Read the model definition and answer for the solid it produces. Units are mm, in the model's axes. Face numbers are marked on the shaded views. A direction names the side the tool comes from. Round coordinates to 2 decimals unless told otherwise and drop trailing zeros. Order: outer loops, then holes, each group sorted by start corner. A loop starts at its lowest first (then second) coordinate and runs counter-clockwise, first axis right, second up. Notation, with made-up numbers: (22.25, 2.25) -> (54.25, 2.25) arc R21 ccw to (54.25, 23.25) -> close; hole circle Ø9 at (16.5, -2). An arc over 180 degrees is marked (long way). Answer as a JSON object with one key per item and string values. Group by question number.
Item 1: Section C-C, the plane y = 215.5 is taken. Write down the section's boundary in (x, z).
Item 2: The mould has two halves that part along Y. Classify the marked faces 1, 2 and 3: pulls with the +Y half, pulls with the -Y half, needs draft (parallel to the pull), parting line crosses it, or undercut.
Item 3: Consider probe 1 along Y at (x, z) = (-66, 7); probe 2 along Z at (x, y) = (-131, 194); probe 3 along Y at (x, z) = (-16, 16.5). Determine where each line is inside the solid, lowest interval first. Write a range as from..to.
Item 4: Given P1, Ø3, axis at x = 66.5, y = 186, coming from the +Z side; P2, Ø8, axis at x = -114, z = 26, coming from the +Y side; P3, Ø10, axis at x = -110.5, z = 7.5, coming from the -Y side, each flat-ended and moving along its own axis, determine where each tip first touches the part or whether it passes through.
Item 5: Section A-A, the plane z = 15 is taken. Count the separate pieces of the cut face and the enclosed holes in it, plus the area to 3 significant figures.
Item 6: For the marked faces 4, 5, 6 and 7, determine the directions among +Z, -Z, +X, -X, +Y, -Y from which every point of the face is accessible in a straight line to the end or side of a thin tool.
Item 7: Section B-B, the plane x = -80.5 is taken. Write down the section's boundary in (y, z), plus the area to 3 significant figures.
Item 8: Section D-D, the plane x = 43.5 is taken. Write down the section's boundary in (y, z).
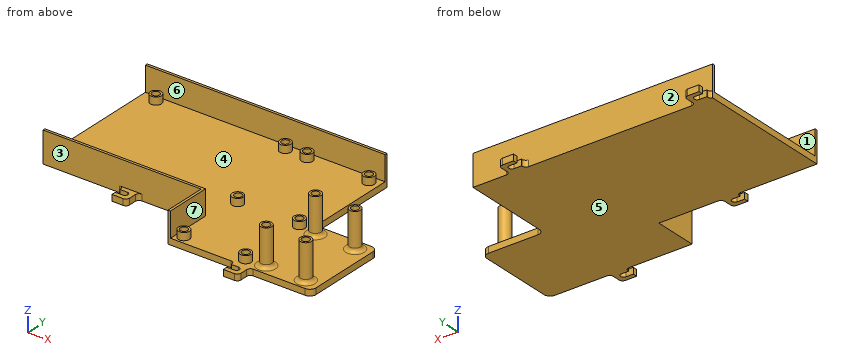
from build123d import *

# Parameters (mm, degrees)
SKETCH1_W            = 128
SKETCH1_H            = 110
SKETCH1_W_2          = 50
SKETCH1_H_2          = 70
BOSS_EXTRUDE1_DEPTH  = 5
SKETCH3_W            = 128
SKETCH3_H            = 2
SKETCH3_W_2          = 194
BOSS_EXTRUDE3_DEPTH  = 20
SKETCH6_W            = 12
SKETCH6_H            = 12
BOSS_EXTRUDE5_DEPTH  = 5
M4_CLEARANCE_HOLE1_D = 4.8
CUT_EXTRUDE1_DEPTH   = 329.83563266
FILLET2_R            = 3
FILLET3_R            = 5
SKETCH15_R           = 4.5
SKETCH15_R_2         = 3.025
BOSS_EXTRUDE6_DEPTH  = 6
SKETCH16_R           = 4.5
SKETCH16_R_2         = 3.025
BOSS_EXTRUDE7_DEPTH  = 30
FILLET4_R            = 3


with BuildPart() as part:
    # Sketch1 → Boss-Extrude1 (new body)
    with BuildSketch(Plane.XY):
        with Locations((-103.32475602, 215.37439567)):
            Rectangle(SKETCH1_W, SKETCH1_H)
        Polygon((26.67524398, 270.37439567), (-39.32475602, 270.37439567), (-39.32475602, 160.37439567), (-39.32475602, 125.37439567), (26.67524398, 125.37439567), (26.67524398, 195.37439567), align=None)
        with Locations((51.67524398, 160.37439567)):
            Rectangle(SKETCH1_W_2, SKETCH1_H_2)
    extrude(amount=BOSS_EXTRUDE1_DEPTH)

    # Sketch3 → Boss-Extrude3 (add)
    with BuildSketch(Plane.XY.offset(5)):
        Polygon((-37.32475602, 162.37439567), (-39.32475602, 162.37439567), (-39.32475602, 160.37439567), (-39.32475602, 125.37439567), (-37.32475602, 125.37439567), align=None)
        with Locations((-103.32475602, 161.37439567)):
            Rectangle(SKETCH3_W, SKETCH3_H)
        with Locations((-70.32475602, 269.37439567)):
            Rectangle(SKETCH3_W_2, SKETCH3_H)
    extrude(amount=BOSS_EXTRUDE3_DEPTH)

    # Sketch6 → Boss-Extrude5 (add)
    with BuildSketch(Plane(origin=(0, 0, 0), x_dir=(-1, 0, 0), z_dir=(0, 0, -1))):
        with Locations((96.32475602, 154.37439567)):
            Rectangle(SKETCH6_W, SKETCH6_H)
        with Locations((159.32475602, 276.37439567)):
            Rectangle(SKETCH6_W, SKETCH6_H)
        with Locations((-20.67524398, 119.37439567)):
            Rectangle(SKETCH6_W, SKETCH6_H)
        with Locations((9.32475602, 276.37439567)):
            Rectangle(SKETCH6_W, SKETCH6_H)
    extrude(amount=-BOSS_EXTRUDE5_DEPTH)

    # M4 Clearance Hole1 (through all)
    with Locations(Plane.XY.offset(5)):
        with Locations((-96.32475602, 154.37439567), (-159.32475602, 276.37439567), (-9.32475602, 276.37439567), (20.67524398, 119.37439567)):
            Hole(M4_CLEARANCE_HOLE1_D / 2)

    # Sketch10 → Cut-Extrude1 (cut, through all)
    with BuildSketch(Plane.XY.offset(5)):
        with BuildLine():
            ThreePointArc((-96.32475602, 151.97439567), (-98.72475602, 154.37439567), (-96.32475602, 156.77439567))
            Line((-96.32475602, 156.77439567), (-102.32475602, 156.77439567))
            Line((-102.32475602, 156.77439567), (-102.32475602, 151.97439567))
            Line((-102.32475602, 151.97439567), (-96.32475602, 151.97439567))
        make_face()
        with BuildLine():
            ThreePointArc((-159.32475602, 273.97439567), (-161.72475602, 276.37439567), (-159.32475602, 278.77439567))
            Line((-159.32475602, 278.77439567), (-165.32475602, 278.77439567))
            Line((-165.32475602, 278.77439567), (-165.32475602, 273.97439567))
            Line((-165.32475602, 273.97439567), (-159.32475602, 273.97439567))
        make_face()
        with BuildLine():
            ThreePointArc((-9.32475602, 273.97439567), (-11.72475602, 276.37439567), (-9.32475602, 278.77439567))
            Line((-9.32475602, 278.77439567), (-15.32475602, 278.77439567))
            Line((-15.32475602, 278.77439567), (-15.32475602, 273.97439567))
            Line((-15.32475602, 273.97439567), (-9.32475602, 273.97439567))
        make_face()
        with BuildLine():
            ThreePointArc((20.67524398, 116.97439567), (18.27524398, 119.37439567), (20.67524398, 121.77439567))
            Line((20.67524398, 121.77439567), (14.67524398, 121.77439567))
            Line((14.67524398, 121.77439567), (14.67524398, 116.97439567))
            Line((14.67524398, 116.97439567), (20.67524398, 116.97439567))
        make_face()
    extrude(amount=-CUT_EXTRUDE1_DEPTH, mode=Mode.SUBTRACT)

    # Fillet2
    # the kernel refuses this fillet: 3 mm, written as the material it adds along each edge
    with BuildSketch(Plane(origin=(-15.32475602, 270.37439567, 0), x_dir=(-1, 0, 0), z_dir=(0, 0, 1)), Plane(origin=(-90.32475602, 160.37439567, 0), x_dir=(1, 0, 0), z_dir=(0, 0, 1))) as fillet2_piece_1:
        with BuildLine():
            CenterArc((FILLET2_R, -FILLET2_R), FILLET2_R, 90, 90)
            Line((0, -FILLET2_R), (0, 0))
            Line((0, 0), (FILLET2_R, 0))
        make_face()
    extrude(amount=5)
    with BuildSketch(Plane(origin=(-3.32475602, 270.37439567, 0), x_dir=(1, 0, 0), z_dir=(0, 0, 1)), Plane(origin=(-102.32475602, 160.37439567, 0), x_dir=(-1, 0, 0), z_dir=(0, 0, 1)), Plane(origin=(-153.32475602, 270.37439567, 0), x_dir=(1, 0, 0), z_dir=(0, 0, 1)), Plane(origin=(14.67524398, 125.37439567, 0), x_dir=(-1, 0, 0), z_dir=(0, 0, 1)), Plane(origin=(26.67524398, 125.37439567, 0), x_dir=(0, -1, 0), z_dir=(0, 0, 1))) as fillet2_piece_2:
        with BuildLine():
            CenterArc((FILLET2_R, FILLET2_R), FILLET2_R, 180, 90)
            Line((0, FILLET2_R), (0, 0))
            Line((0, 0), (FILLET2_R, 0))
        make_face()
    extrude(amount=5)
    with BuildSketch(Plane(origin=(-165.32475602, 270.37439567, 0), x_dir=(-1, 0, 0), z_dir=(0, 0, 1))) as fillet2_piece_3:
        with BuildLine():
            CenterArc((3, -2.828427125), FILLET2_R, 109.471220634, 70.528779366)
            Line((0, -2.828427125), (0, 0))
            Line((0, 0), (2, 0))
        make_face()
    extrude(amount=5)
    # the kernel refuses this fillet: 3 mm, written as the material it takes off along each edge
    with BuildSketch(Plane(origin=(-3.32475602, 282.37439567, -7.5), x_dir=(-1, 0, 0), z_dir=(0, 0, 1)), Plane(origin=(-90.32475602, 148.37439567, -7.5), x_dir=(0, 1, 0), z_dir=(0, 0, 1)), Plane(origin=(-153.32475602, 282.37439567, -7.5), x_dir=(-1, 0, 0), z_dir=(0, 0, 1)), Plane(origin=(26.67524398, 113.37439567, -7.5), x_dir=(0, 1, 0), z_dir=(0, 0, 1))) as fillet2_2_piece_1:
        with BuildLine():
            CenterArc((FILLET2_R, FILLET2_R), FILLET2_R, 180, 90)
            Line((0, FILLET2_R), (0, 0))
            Line((0, 0), (FILLET2_R, 0))
        make_face()
    extrude(amount=20, mode=Mode.SUBTRACT)

    # Fillet3
    fillet3_edges = [part.edges().sort_by_distance(p)[0] for p in [
        (26.67524398, 195.37439567, 2.5),
        (76.67524398, 195.37439567, 2.5),
        (76.67524398, 125.37439567, 2.5),
    ]]
    fillet(fillet3_edges, radius=FILLET3_R)

    # Sketch15 → Boss-Extrude6 (add)
    # profile 1 of 10: a face of its own
    with BuildSketch(Plane.XY.offset(5)):
        with Locations((-154.35475602, 169.52739567)):
            Circle(SKETCH15_R)
        with Locations((-154.35475602, 169.52739567)):
            Circle(SKETCH15_R_2, mode=Mode.SUBTRACT)
    # profile 2 of 10: a face of its own
    with BuildSketch(Plane.XY.offset(5)):
        with Locations((-49.57975602, 262.49139567)):
            Circle(SKETCH15_R)
        with Locations((-49.57975602, 262.49139567)):
            Circle(SKETCH15_R_2, mode=Mode.SUBTRACT)
    # profile 3 of 10: a face of its own
    with BuildSketch(Plane.XY.offset(5)):
        with Locations((-49.57975602, 169.52739567)):
            Circle(SKETCH15_R)
        with Locations((-49.57975602, 169.52739567)):
            Circle(SKETCH15_R_2, mode=Mode.SUBTRACT)
    # profile 4 of 10: a face of its own
    with BuildSketch(Plane.XY.offset(5)):
        with Locations((-31.18175602, 131.55539567)):
            Circle(SKETCH15_R)
        with Locations((-31.18175602, 131.55539567)):
            Circle(SKETCH15_R_2, mode=Mode.SUBTRACT)
    # profile 5 of 10: a face of its own
    with BuildSketch(Plane.XY.offset(5)):
        with Locations((-31.18175602, 188.30539567)):
            Circle(SKETCH15_R)
        with Locations((-30.807769142, 188.30539567)):
            Circle(SKETCH15_R_2, mode=Mode.SUBTRACT)
    # profile 6 of 10: a face of its own
    with BuildSketch(Plane.XY.offset(5)):
        with Locations((18.81824398, 188.30539567)):
            Circle(SKETCH15_R)
        with Locations((18.81824398, 188.30539567)):
            Circle(SKETCH15_R_2, mode=Mode.SUBTRACT)
    # profile 7 of 10: a face of its own
    with BuildSketch(Plane.XY.offset(5)):
        with Locations((18.81824398, 131.55539567)):
            Circle(SKETCH15_R)
        with Locations((18.81824398, 131.55539567)):
            Circle(SKETCH15_R_2, mode=Mode.SUBTRACT)
    # profile 8 of 10: a face of its own
    with BuildSketch(Plane.XY.offset(5)):
        with Locations((-31.18175602, 261.55539567)):
            Circle(SKETCH15_R)
        with Locations((-31.18175602, 261.55539567)):
            Circle(SKETCH15_R_2, mode=Mode.SUBTRACT)
    # profile 9 of 10: a face of its own
    with BuildSketch(Plane.XY.offset(5)):
        with Locations((18.81824398, 261.55539567)):
            Circle(SKETCH15_R)
        with Locations((18.81824398, 261.55539567)):
            Circle(SKETCH15_R_2, mode=Mode.SUBTRACT)
    # profile 10 of 10: a face of its own
    with BuildSketch(Plane.XY.offset(5)):
        with Locations((-154.35475602, 262.49139567)):
            Circle(SKETCH15_R)
        with Locations((-154.35475602, 262.49139567)):
            Circle(SKETCH15_R_2, mode=Mode.SUBTRACT)
    extrude(amount=BOSS_EXTRUDE6_DEPTH)

    # Sketch16 → Boss-Extrude7 (add)
    # profile 1 of 4: a face of its own
    with BuildSketch(Plane.XY.offset(5)):
        with Locations((33.31824398, 134.37439567)):
            Circle(SKETCH16_R)
        with Locations((33.31824398, 134.37439567)):
            Circle(SKETCH16_R_2, mode=Mode.SUBTRACT)
    # profile 2 of 4: a face of its own
    with BuildSketch(Plane.XY.offset(5)):
        with Locations((65.31824398, 134.37439567)):
            Circle(SKETCH16_R)
        with Locations((65.31824398, 134.37439567)):
            Circle(SKETCH16_R_2, mode=Mode.SUBTRACT)
    # profile 3 of 4: a face of its own
    with BuildSketch(Plane.XY.offset(5)):
        with Locations((65.31824398, 186.37439567)):
            Circle(SKETCH16_R)
        with Locations((65.31824398, 186.37439567)):
            Circle(SKETCH16_R_2, mode=Mode.SUBTRACT)
    # profile 4 of 4: a face of its own
    with BuildSketch(Plane.XY.offset(5)):
        with Locations((33.31824398, 186.37439567)):
            Circle(SKETCH16_R)
        with Locations((33.31824398, 186.37439567)):
            Circle(SKETCH16_R_2, mode=Mode.SUBTRACT)
    extrude(amount=BOSS_EXTRUDE7_DEPTH)

    # Fillet4
    fillet4_edges = [part.edges().sort_by_distance(p)[0] for p in [
        (28.81824398, 134.37439567, 5),
        (60.81824398, 134.37439567, 5),
        (60.81824398, 186.37439567, 5),
        (28.81824398, 186.37439567, 5),
    ]]
    fillet(fillet4_edges, radius=FILLET4_R)


solid = part.part
Values found:
{
 "1": {"outline": "(-167.32, 0) -> (26.68, 0) -> (26.68, 5) -> (-167.32, 5) -> close"},
 "2": {"face 1": "undercut", "face 2": "pulls with the +Y half", "face 3": "pulls with the -Y half"},
 "3": {"probe 1": "160.37..162.37, 268.37..270.37", "probe 2": "0..5", "probe 3": "268.37..270.37"},
 "4": {"P1": "z = 5", "P2": "y = 270.37", "P3": "y = 160.37"},
 "5": {"separate pieces": "6", "enclosed holes": "4", "area": "857 mm2"},
 "6": {"face 4": "+Z", "face 5": "-Z, +X, -X, +Y, -Y", "face 6": "+Z, +X, -X", "face 7": "+Z, -Y"},
 "7": {"outline": "(160.37, 0) -> (270.37, 0) -> (270.37, 25) -> (268.37, 25) -> (268.37, 5) -> (162.37, 5) -> (162.37, 25) -> (160.37, 25) -> close", "area": "630 mm2"},
 "8": {"outline": "(125.37, 0) -> (195.37, 0) -> (195.37, 5) -> (125.37, 5) -> close"}
}
